from build123d import *

# Parameters (mm, degrees)
SKETCH_1_R               = 55
EXTRUDE_1_DEPTH          = 8
CUT_EXTRUDE_7_DEPTH      = 358.196024614
HOLE_WIZARD_M5_1_D       = 5.3
PATTERN_CIRCULAR_5_COUNT = 3
CUT_EXTRUDE_2_DEPTH      = 358.196024614
CUT_EXTRUDE_2_DEPTH_BACK = 358.196024614
SKETCH_7_W               = 46
SKETCH_7_H               = 140
CUT_EXTRUDE_4_DEPTH      = 358.196024614
HOLE_WIZARD_M6_1_D       = 6.4
HOLE_WIZARD_M4_1_D       = 3.3
HOLE_WIZARD_M3_1_D       = 3.2
HOLE_WIZARD_9_0_9_1_D    = 9
CUT_EXTRUDE_6_DEPTH      = 10
HOLE_WIZARD_M5_3_D       = 5.5
HOLE_WIZARD_M4_1_2_D     = 4.5


with BuildPart() as part:
    # 草图1 → 凸台-拉伸1 (new body)
    with BuildSketch(Plane(origin=(0, 0, 0), x_dir=(1, 0, 0), z_dir=(0, 1, 0))):
        Polygon((-173.180567757, 192.422381227), (-250, 59.367221574), (-240.170967896, 10.34283858), (-106.041845025, -221.975617006), (-68.5, -255), (68.5, -255), (106.041845025, -221.975617006), (240.170967896, 10.34283858), (250, 59.367221574), (173.180567757, 192.422381227), (129, 230), (-129, 230), align=None)
        with Locations(Location((0, 0, 0), (0, 0, 270))):
            Circle(SKETCH_1_R, mode=Mode.SUBTRACT)
    extrude(amount=EXTRUDE_1_DEPTH)

    # 草图34 → 切除-拉伸7 (cut, through all)
    with BuildSketch(Plane(origin=(0, 8, 0), x_dir=(1, 0, 0), z_dir=(0, 1, 0))):
        Polygon((-144.482648893, 115.748711306), (-128.732648893, 143.028511525), (-183.456761017, 174.623492392), (-242.956761017, 71.566469341), (-188.232648893, 39.971488475), (-172.482648893, 67.251288694), (-124.851251684, 39.751288694), (-96.851251684, 88.248711306), align=None)
        Polygon((172.482648893, 67.251288694), (188.232648893, 39.971488475), (242.956761017, 71.566469341), (183.456761017, 174.623492392), (128.732648893, 143.028511525), (144.482648893, 115.748711306), (96.851251684, 88.248711306), (124.851251684, 39.751288694), align=None)
        Polygon((-28, -183), (-59.5, -183), (-59.5, -255), (59.5, -255), (59.5, -183), (28, -183), (28, -128), (-28, -128), align=None)
    extrude(amount=-CUT_EXTRUDE_7_DEPTH, mode=Mode.SUBTRACT)

    # M5 间隙孔1 (through all)
    with Locations(Plane(origin=(0, 0, 0), x_dir=(-1, 0, 0), z_dir=(0, -1, 0))):
        with Locations((106.225607337, 100.011851027), (137.402521874, 118.011851027), (139.725607337, 41.988148973), (170.902521874, 59.988148973)):
            hole_wizard_m5_1 = Hole(HOLE_WIZARD_M5_1_D / 2)

    # 阵列(圆周)5: M5 间隙孔1 ×3 about axis
    pattern_circular_5_axis = Axis((0, 0, 0), (0, 1, 0))
    for i in range(1, PATTERN_CIRCULAR_5_COUNT):
        add(hole_wizard_m5_1.rotate(pattern_circular_5_axis, i * 360 / PATTERN_CIRCULAR_5_COUNT), mode=Mode.SUBTRACT)

    # 草图5 → 切除-拉伸2 (cut, two sides: drawn at the far end of the back side and taken through both)
    with BuildSketch(Plane(origin=(0, 8, 0), x_dir=(1, 0, 0), z_dir=(0, 1, 0)).offset(-CUT_EXTRUDE_2_DEPTH_BACK)):
        Polygon((35, 145), (120, 230), (-120, 230), (-35, 145), align=None)
    extrude(amount=CUT_EXTRUDE_2_DEPTH + CUT_EXTRUDE_2_DEPTH_BACK, mode=Mode.SUBTRACT)

    # 草图7 → 切除-拉伸4 (cut, through all)
    with BuildSketch(Plane(origin=(0, 8, 0), x_dir=(1, 0, 0), z_dir=(0, 1, 0))):
        with Locations((0, 160)):
            Rectangle(SKETCH_7_W, SKETCH_7_H)
    extrude(amount=-CUT_EXTRUDE_4_DEPTH, mode=Mode.SUBTRACT)

    # M6 间隙孔1 (through all)
    with Locations(Plane(origin=(0, 8, 0), x_dir=(1, 0, 0), z_dir=(0, 1, 0))):
        with Locations((30, 114.64), (-30, 114.64)):
            Hole(HOLE_WIZARD_M6_1_D / 2)

    # Hole Wizard M4 _1 (through all)
    with Locations(Plane(origin=(0, 8, 0), x_dir=(1, 0, 0), z_dir=(0, 1, 0))):
        with Locations((-79, -0.36), (79, -0.36)):
            Hole(HOLE_WIZARD_M4_1_D / 2)

    # 电池座 M3 间隙孔1 (through all)
    with Locations(Plane(origin=(0, 0, 0), x_dir=(-1, 0, 0), z_dir=(0, -1, 0))):
        with Locations((-110.507914412, -66.440289893), (-72.5, -143.903561461), (-134.161542188, -111.623316496), (-48.846372224, -98.720534858)):
            hole_wizard_m3_1 = Hole(HOLE_WIZARD_M3_1_D / 2)

    # Ø9.0 (9) 直径孔1 (through all)
    with Locations(Plane(origin=(0, 0, 0), x_dir=(-1, 0, 0), z_dir=(0, -1, 0))):
        with Locations((-98.248822178, -87.870284237), (-73.442454631, -100.856589683)):
            hole_wizard_9_0_9_1 = Hole(HOLE_WIZARD_9_0_9_1_D / 2)

    # 草图21 → 切除-拉伸6 (cut)
    with BuildSketch(Plane.XZ):
        Polygon((90.903946749, 144.992020949), (96.469506226, 155.623321326), (130.135290754, 137.99904965), (124.569731277, 127.367749272), align=None)
    cut_extrude_6 = extrude(amount=-CUT_EXTRUDE_6_DEPTH, mode=Mode.SUBTRACT)

    # 镜向1: 电池座 M3 间隙孔1, Ø9.0 (9) 直径孔1, 切除-拉伸6 across plane
    add(hole_wizard_m3_1.mirror(Plane(origin=(0, 0, 0), x_dir=(0, 0, 1), z_dir=(1, 0, 0))), mode=Mode.SUBTRACT)
    add(hole_wizard_9_0_9_1.mirror(Plane(origin=(0, 0, 0), x_dir=(0, 0, 1), z_dir=(1, 0, 0))), mode=Mode.SUBTRACT)
    add(cut_extrude_6.mirror(Plane(origin=(0, 0, 0), x_dir=(0, 0, 1), z_dir=(1, 0, 0))), mode=Mode.SUBTRACT)

    # 立柱 M5 间隙孔3 (through all)
    with Locations(Plane(origin=(0, 0, 0), x_dir=(-1, 0, 0), z_dir=(0, -1, 0))):
        with Locations((-237.779820534, 34.02527989), (-222.092017976, 37.170570164), (-138.279747165, 191.912875123), (-148.645986827, 204.100617953), (-89.298360296, -227.381404927), (-78.730557738, -215.368014518)):
            hole_wizard_m5_3 = Hole(HOLE_WIZARD_M5_3_D / 2)

    # 镜向4: 立柱 M5 间隙孔3 across plane
    add(hole_wizard_m5_3.mirror(Plane(origin=(0, 0, 0), x_dir=(0, 0, 1), z_dir=(1, 0, 0))), mode=Mode.SUBTRACT)

    # Hole Wizard M4 _1 2 (through all)
    with Locations(Plane(origin=(0, 0, 0), x_dir=(-1, 0, 0), z_dir=(0, -1, 0))):
        with Locations((128.880701979, 156.505934529), (117.56699348, 167.819643028), (66.655305235, 116.907954782), (77.969013734, 105.594246284), (100.596430732, 133.878517531)):
            hole_wizard_m4_1_2 = Hole(HOLE_WIZARD_M4_1_2_D / 2)

    # 镜向5: Hole Wizard M4 _1 2 across plane
    add(hole_wizard_m4_1_2.mirror(Plane(origin=(0, 0, 0), x_dir=(0, 0, 1), z_dir=(1, 0, 0))), mode=Mode.SUBTRACT)


solid = part.part
Work out the finished part from the listing and answer in its coordinate system (mm). A direction names the side the tool comes from. Coordinates: 2 decimals unless noted, no trailing zeros. Loops run counter-clockwise (first coordinate to the right, second up) from the corner with the lowest first, then second, coordinate; pieces in that order, holes last. Notation, with made-up numbers: (31, 61.25) -> (67, 61.25) arc R22 ccw to (67, 73.25) -> close; hole circle Ø11 at (-29, 39.5). An arc over 180 degrees is marked (long way). Answer as CSV lines item,"result".
1) The part is cut by section B-B (y = 4.75). State how many separate pieces and enclosed holes the cut face has, and give its area (3 significant figures).
A:
separate pieces,"1"
enclosed holes,"53"
area,"118,000 mm²"
2) Straight lines are drawn through the part: probe 1 along Z at (x, y) = (35, 6); probe 2 along Z at (x, y) = (-30, 6.5); probe 3 along Z at (x, y) = (-150, 3.75). For each, find the intervals that lie inside material, in ascending order.
A:
probe 1,"z = -145 to -42.43, 42.43 to 139.82, 144.18 to 175.82, 180.18 to 183"
probe 2,"z = -145 to -117.84, -111.44 to -46.1, 46.1 to 183"
probe 3,"z = -212.14 to -206.49, -201.71 to -155.31, -54.27 to 145.84"
3) The part is cut by section C-C (x = 210.5). Give the vertices of the cut face in (y, z).
A:
outline,"(0, -52.83) -> (8, -52.83) -> (8, 41.05) -> (0, 41.05) -> close"
4) For faces 1 (the face through (-111.047, 4.056, -63.661)), 2 (the face through (151.4, 3.94, -210.95)), 3 (the face through (121, 4.06, -102.19)), 4 (the face through (-215.98, 4.06, -55.99)), 5 (the face through (-120.334, 4.056, -101.806)), determine the directions among +Z, -Z, +X, -X, +Y, -Y from which every point of the face is accessible in a straight line to the end or side of a thin tool.
A:
face 1,"+Y, -Y"
face 2,"-Z, +X, +Y, -Y"
face 3,"+X, +Y, -Y"
face 4,"-Z, +Y, -Y"
face 5,"-X, +Y, -Y"
5) The part is cut by section A-A (z = 195). Give the vertices of the cut face in (x, y).
A:
outline,"(-121.62, 0) -> (-59.5, 0) -> (-59.5, 8) -> (-121.62, 8) -> close; (59.5, 0) -> (121.62, 0) -> (121.62, 8) -> (59.5, 8) -> close"
6) For a pull along Z with two mould halves and no side action, classify faces 6 (the face through (-78, 4, -188)), 7 (the face through (-59, 8, 9)), 8 (the face through (-155.7, 4.1, -158.6)) as released by +Z, released by -Z, zero draft, split by the parting line, or undercut.
A:
face 6,"released by -Z"
face 7,"zero draft"
face 8,"undercut"
7) Flat-ended cylindrical pins translate along their axes: pin 1 (4.5 mm diameter, centred on x = -89.3, z = 227.38, fed in from +Y) (3 decimals); pin 2 (1.5 mm diameter, centred on x = 155, y = 3.5, fed in from +Z); pin 3 (4 mm diameter, centred on x = 103.5, y = 6, fed in from -Z); pin 4 (3 mm diameter, centred on y = 1.5, z = 37, fed in from +X). Find the tip coordinate at first contact, or state that the pin passes through.
A:
pin 1,"passes through"
pin 2,"stops at z = 138.48"
pin 3,"stops at z = -215.5"
pin 4,"stops at x = 213.7"
